Autodesk Inventor part; units mm, degrees
ref_plane "YZ Plane" through (0, 0, 0) normal (1, 0, 0) x (0, 1, 0)
ref_plane "XZ Plane" through (0, 0, 0) normal (0, 1, 0) x (-1, 0, 0)
ref_plane "XY Plane" through (0, 0, 0) normal (0, 0, 1) x (1, 0, 0)
sketch "Sketch1" plane through (0, 0, 0) normal (0, 1, 0) x (-1, 0, 0)
  line L0 (17.3978, -1.9197) -> (-39.6022, -1.9197)
  line L1 (-39.6022, -1.9197) -> (-39.6022, -48.9197)
  line L2 (-39.6022, -48.9197) -> (17.3978, -48.9197)
  line L3 (17.3978, -48.9197) -> (17.3978, -1.9197)
  point P0 (0, 0)
  dimension "d0" = 47
  dimension "d1" = 57
extrude "Extrusion1" add sketch "Sketch1" along normal blind 2
sketch "Sketch2" plane through (0, 2, 0) normal (0, 1, 0) x (1, 0, 0)
  line L0 (-17.3978, 48.9197) -> (-17.3978, 1.9197)
  line L1 (-17.3978, 20.4197) -> (-21.3978, 20.4197)
  line L2 (-24.3978, 23.4197) -> (-24.3978, 27.4197)
  line L3 (-21.3978, 30.4197) -> (-17.3978, 30.4197)
  line L4 (-17.3978, 30.4197) -> (-17.3978, 20.4197)
  line L5 (-17.3978, 1.9197) -> (39.6022, 1.9197)
  arc A0 (-24.3978, 23.4197) -> (-21.3978, 20.4197) centre (-21.3978, 23.4197) ccw
  arc A1 (-21.3978, 30.4197) -> (-24.3978, 27.4197) centre (-21.3978, 27.4197) ccw
  point P0 (0, 0)
  point P1 (-24.3978, 30.4197)
  point P2 (-24.3978, 20.4197)
  dimension "d4" = 10
  dimension "d5" = 18.5
  dimension "d6" = 7
  dimension "d7" = 3
extrude "Extrusion2" add sketch "Sketch2" against normal blind 2
sketch "Sketch3" plane through (0, 2, 0) normal (0, 1, 0) x (1, 0, 0)
  line L0 (39.6022, 1.9197) -> (39.6022, 48.9197)
  line L1 (39.6022, 5.4197) -> (42.6022, 5.4197)
  line L2 (42.6022, 5.4197) -> (42.6022, 45.4197)
  line L3 (42.6022, 45.4197) -> (39.6022, 45.4197)
  line L4 (39.6022, 45.4197) -> (39.6022, 5.4197)
  line L5 (-17.3978, 1.9197) -> (39.6022, 1.9197)
  point P0 (0, 0)
  dimension "d10" = 3
  dimension "d11" = 40
  dimension "d12" = 3.5
extrude "Extrusion3" add sketch "Sketch3" against normal blind 1
fillet "Fillet1" radius 1 2 edges at (42.6022, 1.5, -5.4197) (42.6022, 1.5, -45.4197)
properties part number "BatteryDoor"
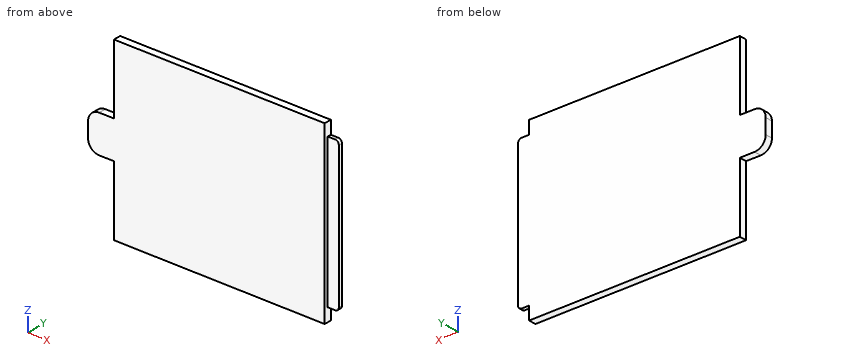
Here's how the part is built. I have some questions about the finished solid (model axes, mm). Coordinates: 2 decimals unless noted, no trailing zeros. Loops run counter-clockwise (first coordinate to the right, second up) from the corner with the lowest first, then second, coordinate; pieces in that order, holes last.
1. For P1, Ø12, axis at x = 15, z = -24.5, coming from the -Y side; P2, Ø2.5, axis at x = 41, z = -25, coming from the -Y side; P3, Ø0.6, axis at x = -18.5, y = 0.5, coming from the -Z side; P4, Ø0.8, axis at x = 40.5, y = 1.5, coming from the -Z side, each with a flat end and sliding along its axis, tell me the tip position at first contact or that it passes through.
2. Imagine slicing it at B-B, the plane y = 1.7. Please give me the cut outline in (x, z), and give its area (3 significant figures).
3. Imagine slicing it at A-A, the plane z = -42.5. Please give me the cut outline in (x, y), and give its area (3 significant figures).
4. Imagine slicing it at D-D, the plane z = -4.5. Please give me the cut outline in (x, y).
5. Imagine slicing it at C-C, the plane z = -25. Please give me the cut outline in (x, y).
6. I need wall thicknesses on L1, parallel to X at y = 0.55, z = -25.5; L2, parallel to X at y = 1.6, z = -34.5. Which ranges of each line are inside material? Lowest first, please.
Taken from the geometry:
1. P1: stops at y = 0
1. P2: stops at y = 1
1. P3: stops at z = -30.42
1. P4: stops at z = -45.42
2. outline: (-24.4, -27.42) arc R3 ccw to (-21.4, -30.42) - (-17.4, -30.42) - (-17.4, -48.92) - (39.6, -48.92) - (39.6, -45.42) - (41.6, -45.42) arc R1 ccw to (42.6, -44.42) - (42.6, -6.42) arc R1 ccw to (41.6, -5.42) - (39.6, -5.42) - (39.6, -1.92) - (-17.4, -1.92) - (-17.4, -20.42) - (-21.4, -20.42) arc R3 ccw to (-24.4, -23.42) - close
2. area: 2,860 mm2
3. outline: (-17.4, 0) - (39.6, 0) - (39.6, 1) - (42.6, 1) - (42.6, 2) - (-17.4, 2) - close
3. area: 117 mm2
4. outline: (-17.4, 0) - (39.6, 0) - (39.6, 2) - (-17.4, 2) - close
5. outline: (-24.4, 0) - (39.6, 0) - (39.6, 1) - (42.6, 1) - (42.6, 2) - (-24.4, 2) - close
6. L1: x = -24.4 to 39.6
6. L2: x = -17.4 to 42.6
